The model under review builds one solid part; all positions refer to its coordinate system, in mm. Face numbers are marked on the shaded views. A direction names the side the tool comes from. Coordinates: 2 decimals unless noted, no trailing zeros. Write each loop counter-clockwise with the first axis right and the second up, starting at its lowest first coordinate (ties: lowest second). Pieces come first, ordered by that corner, then holes. Notation, with made-up numbers: (-14.75, 48.25) - (14.25, 48.25) arc R25 cw to (14.25, 62.25) - close; hole circle Ø2 at (-3, 11). An arc over 180 degrees is marked (long way). Put each result on its own line as item: value. Start each with the question number.
Item 1: Machinability: for the marked faces 4 and 5, which of the approach directions +Z, -Z, +X, -X, +Y, -Y give a long, thin tool a straight path to every point of the face, cutting with its end or side? Answer none if there is none.
Item 2: Consider section B-B on x = -1.5. Give the boundary of the cut face in (y, z), then the cut area to 3 significant figures.
Item 3: Mouldability with a two-part tool opening along Y and no side actions: class the marked faces 1, 2 and 3 as pulls with the +Y half, pulls with the -Y half, needs draft (parallel to the pull), parting line crosses it, or undercut.
Item 4: To check wall thickness, follow L1, parallel to Y at x = 1.75, z = -0.7; L2, parallel to X at y = 0.5, z = -0.45; L3, parallel to X at y = 3.5, z = -0.4. State the ranges of each line that lie inside material, in increasing order. Write a range as [from, to].
Item 5: Consider section D-D on x = 3. Give the boundary of the cut face in (y, z), then the cut area to 3 significant figures.
Item 6: Consider section C-C on z = -0.4. Give the boundary of the cut face in (x, y), then the cut area to 3 significant figures.
Item 7: Consider section A-A on y = 0. Give the boundary of the cut face in (x, z), then the cut area to 3 significant figures.
Item 8: For pin 1 (1.5 mm diameter, centred on x = 0.5, y = 1, fed in from -Z), flat-tipped, find the tip position at first contact; note if it passes through.
```python
from build123d import *

# Parameters (mm, degrees)
ESQUISSE1_R             = 6.835577951
ESQUISSE1_R_2           = 2.45
BOSS_EXTRU_1_DEPTH      = 0.8
ESQUISSE3_R             = 0.85
ENL_V_MAT_EXTRU_1_DEPTH = 10.700012982


with BuildPart() as part:
    # Esquisse1 → Boss.-Extru.1 (new body)
    with BuildSketch(Plane.XY):
        Circle(ESQUISSE1_R)
        Circle(ESQUISSE1_R_2, mode=Mode.SUBTRACT)
    extrude(amount=-BOSS_EXTRU_1_DEPTH)

    # Esquisse3 → Enlèv. mat.-Extru.1 (cut, through all)
    with BuildSketch(Plane(origin=(0, 0, -0.8), x_dir=(-1, 0, 0), z_dir=(0, 0, -1))):
        with Locations((-0.129516777, 2.99720293)):
            Circle(ESQUISSE3_R)
        with Locations((0.129516777, -2.99720293)):
            Circle(ESQUISSE3_R)
    extrude(amount=-ENL_V_MAT_EXTRU_1_DEPTH, mode=Mode.SUBTRACT)


solid = part.part
```
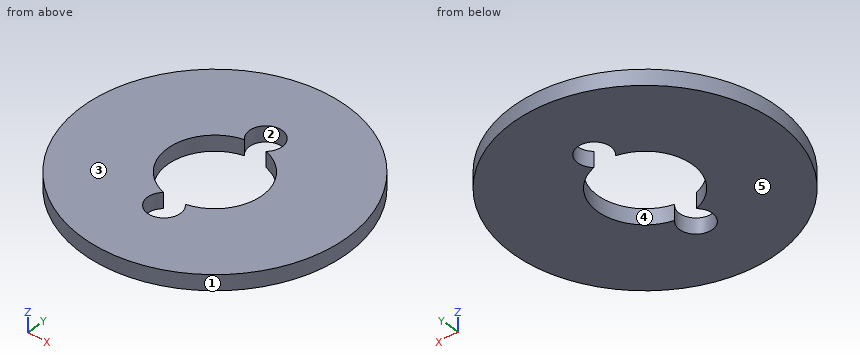
Report:
1. face 4: +Z, -Z
1. face 5: -Z, +X, -X, +Y, -Y
2. outline: (-6.67, -0.8) - (-1.94, -0.8) - (-1.94, 0) - (-6.67, 0) - close; (1.94, -0.8) - (6.67, -0.8) - (6.67, 0) - (1.94, 0) - close
2. area: 7.57 mm²
3. face 1: parting line crosses it
3. face 2: undercut
3. face 3: needs draft
4. L1: [-6.61, -1.71], [1.71, 6.61]
4. L2: [-6.82, -2.4], [2.4, 6.82]
4. L3: [-5.87, -0.56], [0.81, 5.87]
5. outline: (-6.14, -0.8) - (6.14, -0.8) - (6.14, 0) - (-6.14, 0) - close
5. area: 9.83 mm²
6. outline: circle Ø13.67 at (0, 0); hole (-0.68, -2.35) arc R0.85 ccw (long way) to (0.48, -2.4) arc R2.45 ccw to (0.68, 2.35) arc R0.85 ccw (long way) to (-0.48, 2.4) arc R2.45 ccw to start
6. area: 124 mm²
7. outline: (-6.84, -0.8) - (-2.45, -0.8) - (-2.45, 0) - (-6.84, 0) - close; (2.45, -0.8) - (6.84, -0.8) - (6.84, 0) - (2.45, 0) - close
7. area: 7.02 mm²
8. pin 1: through
